from build123d import *

# Parameters (mm, degrees)
SKETCH1_W           = 250
SKETCH1_H           = 123
SKETCH1_W_2         = 13.5
SKETCH1_H_2         = 13.5
BOSS_EXTRUDE1_DEPTH = 2
SKETCH3_W           = 250
SKETCH3_H           = 123
SKETCH3_W_2         = 141.095287024
SKETCH3_H_2         = 84.970220395
CUT_EXTRUDE2_DEPTH  = 62
SKETCH4_R           = 1
CUT_EXTRUDE3_DEPTH  = 62


with BuildPart() as part:
    # Sketch1 → Boss-Extrude1 (new body)
    with BuildSketch(Plane(origin=(0, 0, 0), x_dir=(-1, 0, 0), z_dir=(0, 0, 1))):
        Rectangle(SKETCH1_W, SKETCH1_H)
        with Locations((92, -31.5)):
            Rectangle(SKETCH1_W_2, SKETCH1_H_2, mode=Mode.SUBTRACT)
        with Locations((92, -1.5)):
            Rectangle(SKETCH1_W_2, SKETCH1_H_2, mode=Mode.SUBTRACT)
        with Locations((62, -41.5)):
            Rectangle(SKETCH1_W_2, SKETCH1_H_2, mode=Mode.SUBTRACT)
        with Locations((62, -11.5)):
            Rectangle(SKETCH1_W_2, SKETCH1_H_2, mode=Mode.SUBTRACT)
        with Locations((32, -41.5)):
            Rectangle(SKETCH1_W_2, SKETCH1_H_2, mode=Mode.SUBTRACT)
        with Locations((32, -11.5)):
            Rectangle(SKETCH1_W_2, SKETCH1_H_2, mode=Mode.SUBTRACT)
        with Locations((2, -26.5)):
            Rectangle(SKETCH1_W_2, SKETCH1_H_2, mode=Mode.SUBTRACT)
        with Locations((2, 3.5)):
            Rectangle(SKETCH1_W_2, SKETCH1_H_2, mode=Mode.SUBTRACT)
    extrude(amount=BOSS_EXTRUDE1_DEPTH)

    # Sketch3 → Cut-Extrude2 (cut)
    with BuildSketch(Plane.XY.offset(2)):
        Rectangle(SKETCH3_W, SKETCH3_H)
        with Locations((-43.596913119, 14.422576882)):
            Rectangle(SKETCH3_W_2, SKETCH3_H_2, mode=Mode.SUBTRACT)
    extrude(amount=-CUT_EXTRUDE2_DEPTH, mode=Mode.SUBTRACT)

    # Sketch4 → Cut-Extrude3 (cut)
    with BuildSketch(Plane.XY.offset(2)):
        with Locations((23.950730393, -25.062533315)):
            Circle(SKETCH4_R)
        with Locations((23.950730393, 53.90768708)):
            Circle(SKETCH4_R)
        with Locations((-111.144556631, 53.90768708)):
            Circle(SKETCH4_R)
        with Locations((-111.144556631, -25.062533315)):
            Circle(SKETCH4_R)
    extrude(amount=-CUT_EXTRUDE3_DEPTH, mode=Mode.SUBTRACT)


solid = part.part
The model under review builds one solid part; all positions refer to its coordinate system, in mm. Coordinates: 2 decimals unless noted, no trailing zeros. Loops run counter-clockwise (first coordinate to the right, second up) from the corner with the lowest first, then second, coordinate; pieces in that order, holes last. Notation, with made-up numbers: M -22.75,-15.5 L 35.25,-15.5 A12 cw 35.25,-9.5 Z; hole C 28,70 d7. An arc over 180 degrees is marked long. Put each result on its own line as item: value. Start each with the question number.
Q1. Wall thickness on line 1 (Y direction, x = -89.5, z = 0.7); line 2 (X direction, y = 26, z = 1.3); line 3 (X direction, y = 15, z = 1.8): over which ranges is each line inside the solid? List them lowest first.
Q2. Add section A-A (y = 16.5). Write out the cut boundary in (x, z), and give its area (3 significant figures).
Q3. The part is to be moulded in two halves that separate along Z. For faces 1 (the flat face through (-43, 14, 2)), 2 (the flat face through (-43, 14, 0)), say which applies: +Z half, -Z half, draft (parallel to the pull), parting line (faces both ways), or undercut.
Q4. Add section B-B (x = -3.5). Write out the cut boundary in (y, z), and give its area (3 significant figures).
Q5. Add section C-C (z = 0.7). Count the separate pieces of the cut face and the enclosed holes in it, and give its area (3 significant figures).
Answers:
1. line 1: y = -28.06 to -5.25, 8.25 to 24.75, 38.25 to 56.91
1. line 2: x = -114.14 to -98.75, -85.25 to -8.75, 4.75 to 26.95
1. line 3: x = -114.14 to -68.75, -55.25 to -38.75, -25.25 to 26.95
2. outline: M -114.14,0 L -68.75,0 L -68.75,2 L -114.14,2 Z; M -55.25,0 L -38.75,0 L -38.75,2 L -55.25,2 Z; M -25.25,0 L 26.95,0 L 26.95,2 L -25.25,2 Z
2. area: 228 mm^2
3. face 1: +Z half
3. face 2: -Z half
4. outline: M -28.06,0 L -10.25,0 L -10.25,2 L -28.06,2 Z; M 3.25,0 L 19.75,0 L 19.75,2 L 3.25,2 Z; M 33.25,0 L 56.91,0 L 56.91,2 L 33.25,2 Z
4. area: 116 mm^2
5. separate pieces: 1
5. enclosed holes: 12
5. area: 10,500 mm^2
